from build123d import *

# Parameters (mm, degrees)
F0_R     = 10.16
F0_R_2   = 6.985
F1_DEPTH = 31.75
F2_R     = 8.255
F2_R_2   = 6.985
F3_DEPTH = 10.16
F4_R     = 6.985
F4_R_2   = 4.445
F5_DEPTH = 10.16


with BuildPart() as f1:
    # F0 (on Top) → F1 (new body)
    with BuildSketch(Plane.XY):
        Circle(F0_R)
        Circle(F0_R_2, mode=Mode.SUBTRACT)
    extrude(amount=F1_DEPTH)

    # F2 (on face) → F3 (join)
    with BuildSketch(Plane.XY.offset(31.75)):
        Circle(F2_R)
        Circle(F2_R_2, mode=Mode.SUBTRACT)
    extrude(amount=F3_DEPTH)

    # F4 (on face) → F5 (join)
    with BuildSketch(Plane(origin=(0, 0, 0), x_dir=(1, 0, 0), z_dir=(0, 0, -1))):
        Circle(F4_R)
        Circle(F4_R_2, mode=Mode.SUBTRACT)
    extrude(amount=-F5_DEPTH)


solid = f1.part
Geometry check sheet. Reference: the model listing, model coordinates, mm. A direction names the side the tool comes from. Give positions to 0.01 mm unless a question says otherwise; leave off trailing zeros. Loops run counter-clockwise (first coordinate to the right, second up) from the corner with the lowest first, then second, coordinate; pieces in that order, holes last. Notation, with made-up numbers: (-0.5, 83.5) -> (11.5, 83.5) arc R21 ccw to (11.5, 92.5) -> close; hole circle Ø9 at (69.25, 13). An arc over 180 degrees is marked (long way). Answer in a Markdown table with one row per item. Add a question column.
1) Draft check along Y on faces 1 (the face through (-0.909, 6.926, 25.813)), 2 (the face through (-7, 2, 41.91)), 3 (the face through (7.874, 2.48, 36.759)). Enter one of: pulls with the +Y half, pulls with the -Y half, needs draft (parallel to the pull), parting line crosses it, or undercut.
2) Set-up check for faces 4 (the face through (-1.323, 10.074, 15.653)), 5 (the face through (0, 5, 10.16)): record each of +Z, -Z, +X, -X, +Y, -Y from which the full face is reachable in a straight line by a thin tool's end or side.
3) Material ranges on probe 1 along Y at (x, z) = (0, 6.5) (3 decimals); probe 2 along Y at (x, z) = (0, 27.5) (3 decimals); probe 3 along Z at (x, y) = (0.25, -6.5), recorded low to high. Write a range as from..to.
4) Gauge pin test, flat ends, axial feed: P1, Ø7, axis at x = -2.5, y = 1, coming from the +Z side; P2, Ø12, axis at x = -7.5, y = 0, coming from the -Z side; P3, Ø4, axis at y = -4.5, z = 6, coming from the +X side; P4, Ø1, axis at x = 3.5, z = 20.5, coming from the +Y side. Record the tip position at first contact, or that the pin passes through.
5) Cross-section at A-A on y = 0. Record the boundary of the cut face in (x, z) (3 decimals), and give its area (3 significant figures).
6) Cross-section at C-C on z = 9.5. Record the boundary of the cut face in (x, y) (3 decimals), and give its area (3 significant figures).
7) Cross-section at D-D on x = 5. Record the boundary of the cut face in (y, z).
Outcome:
| question | item | result |
|---|---|---|
| 1 | face 1 | undercut |
| 1 | face 2 | needs draft |
| 1 | face 3 | parting line crosses it |
| 2 | face 4 | +Z, -Z |
| 2 | face 5 | +Z |
| 3 | probe 1 | y = -10.16..-4.445, 4.445..10.16 |
| 3 | probe 2 | y = -10.16..-6.985, 6.985..10.16 |
| 3 | probe 3 | z = 0..10.16 |
| 4 | P1 | stops at z = 10.16 |
| 4 | P2 | stops at z = 0 |
| 4 | P3 | stops at x = 9.85 |
| 4 | P4 | stops at y = 9.71 |
| 5 | outline | (-10.16, 0) -> (-4.445, 0) -> (-4.445, 10.16) -> (-6.985, 10.16) -> (-6.985, 41.91) -> (-8.255, 41.91) -> (-8.255, 31.75) -> (-10.16, 31.75) -> close; (4.445, 0) -> (10.16, 0) -> (10.16, 31.75) -> (8.255, 31.75) -> (8.255, 41.91) -> (6.985, 41.91) -> (6.985, 10.16) -> (4.445, 10.16) -> close |
| 5 | area | 279 mm^2 |
| 6 | outline | circle Ø20.32 at (0, 0); hole circle Ø8.89 at (0, 0) |
| 6 | area | 262 mm^2 |
| 7 | outline | (-8.84, 0) -> (8.84, 0) -> (8.84, 31.75) -> (6.57, 31.75) -> (6.57, 41.91) -> (4.88, 41.91) -> (4.88, 10.16) -> (-4.88, 10.16) -> (-4.88, 41.91) -> (-6.57, 41.91) -> (-6.57, 31.75) -> (-8.84, 31.75) -> close |
